from build123d import *

# Parameters (mm, degrees)
SKETCH1_W                = 310
SKETCH1_H                = 280
SKETCH1_W_2              = 270
SKETCH1_H_2              = 240
BOSS_EXTRUDE1_DEPTH      = 4
BOSS_EXTRUDE3_DEPTH      = 16
BOSS_EXTRUDE3_DEPTH_BACK = 4
SKETCH2_W                = 270
SKETCH2_H                = 240
SKETCH2_W_2              = 263.25
SKETCH2_H_2              = 234
SKETCH4_W                = 263.25
SKETCH4_H                = 234
BOSS_EXTRUDE4_DEPTH      = 4
SKETCH6_W                = 20
SKETCH6_H                = 3
SKETCH6_W_2              = 10
SKETCH6_H_2              = 2
BOSS_EXTRUDE5_DEPTH      = 10
SKETCH7_W                = 3
SKETCH7_H                = 20
BOSS_EXTRUDE6_DEPTH      = 10
FILLET1_R                = 10


with BuildPart() as part:
    # Sketch1 → Boss-Extrude1 (new body)
    with BuildSketch(Plane.XY):
        Rectangle(SKETCH1_W, SKETCH1_H)
        Rectangle(SKETCH1_W_2, SKETCH1_H_2, mode=Mode.SUBTRACT)
    extrude(amount=BOSS_EXTRUDE1_DEPTH)

    # Sketch2 → Boss-Extrude3 (add, two sides: drawn at the far end of the back side and taken through both)
    with BuildSketch(Plane.XY.offset(4).offset(-BOSS_EXTRUDE3_DEPTH_BACK)):
        Rectangle(SKETCH2_W, SKETCH2_H)
        Rectangle(SKETCH2_W_2, SKETCH2_H_2, mode=Mode.SUBTRACT)
    extrude(amount=BOSS_EXTRUDE3_DEPTH + BOSS_EXTRUDE3_DEPTH_BACK)

    # Sketch4 → Boss-Extrude4 (add)
    with BuildSketch(Plane.XY.offset(20)):
        Rectangle(SKETCH4_W, SKETCH4_H)
    extrude(amount=-BOSS_EXTRUDE4_DEPTH)

    # Sketch6 → Boss-Extrude5 (add)
    with BuildSketch(Plane.XY.offset(4)):
        with Locations((-145, 83.5)):
            Rectangle(SKETCH6_W, SKETCH6_H)
        with Locations((145, 93.5)):
            Rectangle(SKETCH6_W, SKETCH6_H)
        with Locations((145, -93.5)):
            Rectangle(SKETCH6_W, SKETCH6_H)
        with Locations((-145, -83.5)):
            Rectangle(SKETCH6_W, SKETCH6_H)
        with Locations((-140, -119)):
            Rectangle(SKETCH6_W_2, SKETCH6_H_2)
        with Locations((-140, 119)):
            Rectangle(SKETCH6_W_2, SKETCH6_H_2)
    extrude(amount=BOSS_EXTRUDE5_DEPTH)

    # Sketch7 → Boss-Extrude6 (add)
    with BuildSketch(Plane.XY.offset(4)):
        with Locations((-136.5, 130)):
            Rectangle(SKETCH7_W, SKETCH7_H)
        with Locations((-74.5, 130)):
            Rectangle(SKETCH7_W, SKETCH7_H)
        with Locations((-136.5, -130)):
            Rectangle(SKETCH7_W, SKETCH7_H)
        with Locations((-74.5, -130)):
            Rectangle(SKETCH7_W, SKETCH7_H)
    extrude(amount=BOSS_EXTRUDE6_DEPTH)

    # Fillet1
    # the kernel refuses this fillet: 10 mm, written as the material it adds along each edge
    with BuildSketch(Plane(origin=(-138, -120, 4), x_dir=(-1, 0, 0), z_dir=(0, 0, 1))) as fillet1_piece_1:
        with BuildLine():
            CenterArc((10, 9.539392014), FILLET1_R, 180, 72.542396876)
            Line((0, 9.539392014), (-0.2, 9.539392014))
            Line((-0.2, 9.539392014), (-0.2, 0))
            Line((-0.2, 0), (0, -0.2))
            ThreePointArc((0, -0.2), (3.5, -0.2), (6.94, -0.19078784))
            Line((6.94, -0.19078784), (7, 0))
        make_face()
    extrude(amount=10)
    with BuildSketch(Plane(origin=(-138, 120, 4), x_dir=(0, 1, 0), z_dir=(0, 0, 1))) as fillet1_piece_2:
        with BuildLine():
            CenterArc((9.539392014, 10), FILLET1_R, 197.457603124, 72.542396876)
            Line((0, 7), (-0.19078784, 6.94))
            ThreePointArc((-0.19078784, 6.94), (-0.2, 3.5), (-0.2, 0))
            Line((-0.2, 0), (0, -0.2))
            Line((0, -0.2), (9.539392014, -0.2))
            Line((9.539392014, -0.2), (9.539392014, 0))
        make_face()
    extrude(amount=10)


solid = part.part
Source: CAD feature listing. Evaluate the final solid. Frame: model axes, mm. A direction names the side the tool comes from. Give positions to 0.01 mm unless a question says otherwise; leave off trailing zeros. Write each loop counter-clockwise with the first axis right and the second up, starting at its lowest first coordinate (ties: lowest second). Pieces come first, ordered by that corner, then holes. Notation, with made-up numbers: (-25.75, 5) -> (-20.75, 5) arc R18 ccw to (-20.75, 11) -> close; hole circle Ø8 at (0, -21). An arc over 180 degrees is marked (long way). Return JSON: item names as keys, results as strings. Group by question number.
1. Pin query (flat end, axial travel): pin 1 Ø5 at (x, y) = (-141, 128) entering from +Z; pin 2 Ø2 at (y, z) = (119, 11) entering from -X; pin 3 Ø5 at (y, z) = (-52.5, 11.5) entering from -X. Return the tip coordinate at first contact, or that it passes through.
2. Section B-B, the plane x = -61. Output: boundary loops of the cut face in (y, z).
3. Material intervals for line 1 (Y direction, x = -67, z = 8.75); line 2 (X direction, y = -1, z = 4.75) (3 decimals); line 3 (X direction, y = 18, z = 1.5) (3 decimals), sorted ascending. Write a range as from..to.
4. Access query for faces 4 (the face through (-73, 130, 9)), 5 (the face through (-140, 118, 9)), 6 (the face through (-73, -130, 9)), 7 (the face through (-138, -135, 9)), 8 (the face through (-106, -130, 4)). Directions: +Z, -Z, +X, -X, +Y, -Y. A direction counts if a zero-diameter tool reaches every point of the face in a straight line with its end or side. Return the directions, or none.
5. Section A-A, the plane y = -73.5. Output: boundary loops of the cut face in (x, z) (3 decimals), then the cut area to 3 significant figures.
6. Mould query, pull axis Y, two halves, no side actions, for faces 1 (the face through (-2, -122, 0)), 2 (the face through (145, -92, 9)), 3 (the face through (-139.89, -123.69, 8.93)). Classes: +Y half, -Y half, draft (parallel to the pull), parting line (faces both ways), or undercut.
Determined:
{
 "1": {"pin 1": "stops at z = 4", "pin 2": "stops at x = -145", "pin 3": "stops at x = -135"},
 "2": {"outline": "(-140, 0) -> (-117, 0) -> (-117, 16) -> (117, 16) -> (117, 0) -> (140, 0) -> (140, 4) -> (120, 4) -> (120, 20) -> (-120, 20) -> (-120, 4) -> (-140, 4) -> close"},
 "3": {"line 1": "y = -120..-117, 117..120", "line 2": "x = -135..-131.625, 131.625..135", "line 3": "x = -155..-131.625, 131.625..155"},
 "4": {"face 4": "+Z, +X, +Y", "face 5": "+Z, -X", "face 6": "+Z, +X, -Y", "face 7": "+Z, -X, -Y", "face 8": "+Z, -Y"},
 "5": {"outline": "(-155, 0) -> (-131.625, 0) -> (-131.625, 16) -> (131.625, 16) -> (131.625, 0) -> (155, 0) -> (155, 4) -> (135, 4) -> (135, 20) -> (-135, 20) -> (-135, 4) -> (-155, 4) -> close", "area": "1,350 mm2"},
 "6": {"face 1": "draft", "face 2": "undercut", "face 3": "-Y half"}
}
